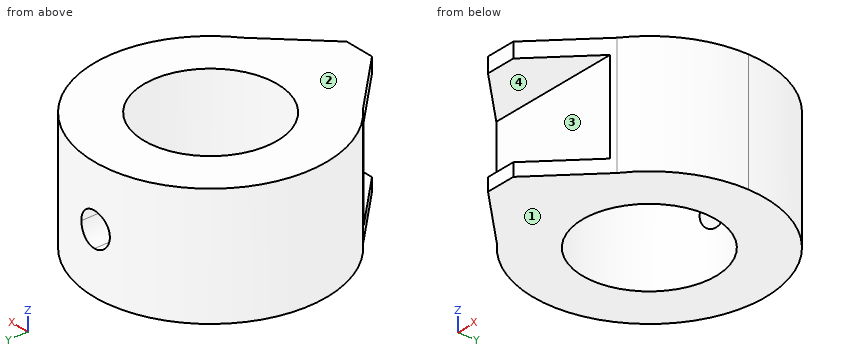
from build123d import *

# Parameters (mm, degrees)
F0_R     = 6.725
F1_DEPTH = 12
F4_DEPTH = 10
F5_W     = 3
F5_H     = 9.2
F5_W_2   = 6.6256758422
F6_DEPTH = 5.3


with BuildPart() as f1:
    # F0 (on Top) → F1 (new body)
    with BuildSketch(Plane.XY):
        with BuildLine():
            ThreePointArc((7.1251998651, -9.3116675135), (10.5123402109, -5.1929113502), (11.725, 0))
            ThreePointArc((11.725, 0), (-5.1929113502, 10.5123402109), (-7.1251998651, -9.3116675135))
            ThreePointArc((-7.1251998651, -9.3116675135), (0, -11.725), (7.1251998651, -9.3116675135))
        make_face()
        Circle(F0_R, mode=Mode.SUBTRACT)
        with BuildLine():
            ThreePointArc((7.1251998651, -9.3116675135), (0, -11.725), (-7.1251998651, -9.3116675135))
            Line((-7.1251998651, -9.3116675135), (-1.5, -15))
            Line((-1.5, -15), (0, -15))
            Line((0, -15), (1.5, -15))
            Line((1.5, -15), (7.1251998651, -9.3116675135))
        make_face()
    extrude(amount=F1_DEPTH)

    # F3 (on offset) → F4 (cut)
    with BuildSketch(Plane.XZ.offset(-12)):
        with BuildLine():
            ThreePointArc((0, 7.6875), (-1.6875, 6), (0, 4.3125))
            Line((0, 4.3125), (0, 7.6875))
        make_face()
        with BuildLine():
            Line((0, 7.6875), (0, 4.3125))
            ThreePointArc((0, 4.3125), (1.1932426933, 4.8067573067), (1.6875, 6))
            ThreePointArc((1.6875, 6), (1.1932426933, 7.1932426933), (0, 7.6875))
        make_face()
    extrude(amount=F4_DEPTH, mode=Mode.SUBTRACT)

    # F5 (on face) → F6 (cut)
    with BuildSketch(Plane.XZ.offset(15)):
        with Locations((0, 5.9)):
            Rectangle(F5_W, F5_H)
        with Locations((-4.8128379211, 5.9)):
            Rectangle(F5_W_2, F5_H)
        with Locations((4.8128379211, 5.9)):
            Rectangle(F5_W_2, F5_H)
    extrude(amount=-F6_DEPTH, mode=Mode.SUBTRACT)


solid = f1.part
Design review of the part built by this model. Coordinates are the model's own, in mm. Face numbers are marked on the shaded views. Give positions to 0.01 mm unless a question says otherwise; leave off trailing zeros. Write each loop counter-clockwise with the first axis right and the second up, starting at its lowest first coordinate (ties: lowest second). Pieces come first, ordered by that corner, then holes. Notation, with made-up numbers: M -31.75,85 L -20.75,85 A23 ccw -20.75,95 Z; hole C 15,30 d4. An arc over 180 degrees is marked long. Return JSON: item names as keys, results as strings. Group by question number.
Item 1: The part is to be moulded in two halves that separate along Z. For the marked faces 1, 2, 3 and 4, say which applies: pulls with the +Z half, pulls with the -Z half, needs draft (parallel to the pull), parting line crosses it, or undercut.
Item 2: Take a section at D-D (z = 11.25). Give the boundary of the cut face in (x, y) (3 decimals).
Item 3: Take a section at B-B (y = -3). Give the boundary of the cut face in (x, z).
Item 4: Take a section at A-A (z = 2.5). Give the boundary of the cut face in (x, y) (3 decimals).
Item 5: Clearance check with flat-ended pins moving along their axes: pin 1 Ø1.5 at (y, z) = (2, 5) entering from +X; pin 2 Ø1.5 at (x, z) = (2.5, 4) entering from -Y. State where each tip first meets the part, or that it passes through.
Item 6: Wall thickness on line 1 along Y through (x, z) = (0, 3) (3 decimals); line 2 along X through (y, z) = (3.75, 4); line 3 along Y through (x, z) = (0, 6.75) (3 decimals): over which ranges is each line inside the solid? List them lowest first.
Item 7: Take a section at C-C (x = -2.5). Give the boundary of the cut face in (y, z).
Return value:
{
 "1": {"face 1": "pulls with the -Z half", "face 2": "pulls with the +Z half", "face 3": "undercut", "face 4": "undercut"},
 "2": {"outline": "M -7.125,-9.312 L -1.5,-15 L 1.5,-15 L 7.125,-9.312 A11.725 ccw long Z; hole C 0,0 d13.45"},
 "3": {"outline": "M -11.33,0 L -6.02,0 L -6.02,12 L -11.33,12 Z; M 6.02,0 L 11.33,0 L 11.33,12 L 6.02,12 Z"},
 "4": {"outline": "M -7.125,-9.312 L -6.741,-9.7 L 6.741,-9.7 L 7.125,-9.312 A11.725 ccw long Z; hole C 0,0 d13.45"},
 "5": {"pin 1": "stops at x = 11.66", "pin 2": "stops at y = -9.7"},
 "6": {"line 1": "y = -9.7 to -6.725, 6.725 to 11.725", "line 2": "x = -11.11 to -5.58, 5.58 to 11.11", "line 3": "y = -9.7 to -6.725"},
 "7": {"outline": "M -13.99,0 L -6.24,0 L -6.24,12 L -13.99,12 L -13.99,10.5 L -9.7,10.5 L -9.7,1.3 L -13.99,1.3 Z; M 6.24,0 L 11.46,0 L 11.46,12 L 6.24,12 Z"}
}
